```python
from build123d import *

# Parameters (mm, degrees)
SKETCH1_W               = 45.72
SKETCH1_H               = 17.78
BOSS_EXTRUDE1_DEPTH     = 45.72
SKETCH2_W               = 38.1
SKETCH2_H               = 12.7
CUT_EXTRUDE1_DEPTH      = 41.91
SKETCH6_R               = 3.048
CUT_EXTRUDE2_DEPTH      = 9.328339826
CUT_EXTRUDE2_DEPTH_BACK = 15.24


with BuildPart() as part:
    # Sketch1 → Boss-Extrude1 (new body)
    with BuildSketch(Plane(origin=(0, 0, 0), x_dir=(1, 0, 0), z_dir=(0, 1, 0))):
        with Locations((22.86, 8.89)):
            Rectangle(SKETCH1_W, SKETCH1_H)
    extrude(amount=BOSS_EXTRUDE1_DEPTH)

    # Sketch2 → Cut-Extrude1 (cut)
    with BuildSketch(Plane(origin=(0, 45.72, 0), x_dir=(1, 0, 0), z_dir=(0, 1, 0))):
        with Locations((22.86, 8.89)):
            Rectangle(SKETCH2_W, SKETCH2_H)
    extrude(amount=-CUT_EXTRUDE1_DEPTH, mode=Mode.SUBTRACT)

    # Sketch6 → Cut-Extrude2 (cut, two sides)
    with BuildSketch(Plane(origin=(0, 0, 0), x_dir=(0.974501657, 0.176548089, -0.138482102), z_dir=(0.182159664, -0.982845594, 0.028851256))) as cut_extrude2_sk:
        with Locations((23.128298386, -5.852866773)):
            Circle(SKETCH6_R)
        with Locations((16.079712461, -6.800485078)):
            Circle(SKETCH6_R)
        with Locations((30.176884312, -4.905248468)):
            Circle(SKETCH6_R)
    extrude(amount=CUT_EXTRUDE2_DEPTH, mode=Mode.SUBTRACT)
    extrude(cut_extrude2_sk.sketch, amount=-CUT_EXTRUDE2_DEPTH_BACK, mode=Mode.SUBTRACT)


solid = part.part
```
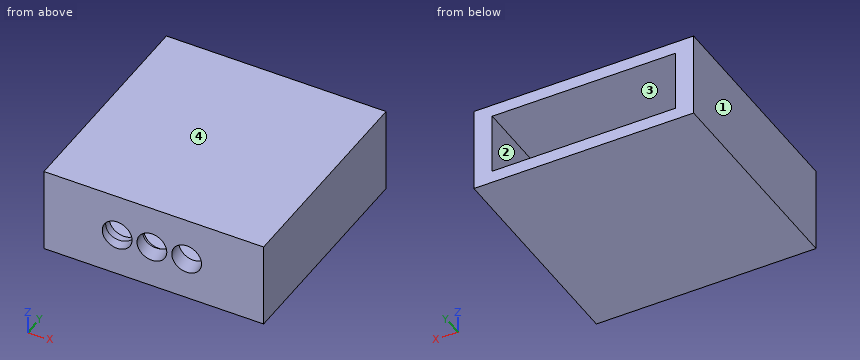
Model file for the job. Use its own axes, mm. Face numbers are marked on the shaded views. Coordinates: 2 decimals unless noted, no trailing zeros. Order: outer loops, then holes, each group sorted by start corner. A loop starts at its lowest first (then second) coordinate and runs counter-clockwise, first axis right, second up. Notation, with made-up numbers: (62, 11.25) - (95, 11.25) arc R12 cw to (95, 28.25) - close; hole circle Ø2 at (57, 84.25). An arc over 180 degrees is marked (long way). Return JSON: item names as keys, results as strings. Group by question number.
1) Saw through at A-A, the plane y = 42. Write the cut outline in (x, z).
2) Flat gauge pins, fed straight in: P1, Ø1, axis at x = 41, z = -3.5, coming from the -Y side; P2, Ø1, axis at x = 5.5, z = -4, coming from the +Y side. Where does each tip first touch, or does it go through?
3) Saw through at C-C, the plane z = -8.5. Count the separate pieces of the cut face and the enclosed holes in it, plus the area to 3 significant figures.
4) Saw through at B-B, the plane z = -13. Write the cut outline in (x, y), plus the area to 3 significant figures.
5) Mould opens along X. For the marked faces 1, 2, 3 and 4 say: released by +X, released by -X, zero draft, split by the parting line, or undercut.
6) Probe line 1 (Z direction, x = 7, y = 41.5); line 2 (X direction, y = 18, z = -10.5); line 3 (Y direction, x = 30, z = -12). List the from-to ranges inside material, lowest first. Write a range as from..to.
Values found:
{
 "1": {"outline": "(0, -17.78) - (45.72, -17.78) - (45.72, 0) - (0, 0) - close; hole (3.81, -15.24) - (41.91, -15.24) - (41.91, -2.54) - (3.81, -2.54) - close"},
 "2": {"P1": "stops at y = 0", "P2": "stops at y = 3.81"},
 "3": {"separate pieces": "4", "enclosed holes": "0", "area": "423 mm²"},
 "4": {"outline": "(0, 0) - (45.72, 0) - (45.72, 45.72) - (41.91, 45.72) - (41.91, 3.81) - (3.81, 3.81) - (3.81, 45.72) - (0, 45.72) - close", "area": "494 mm²"},
 "5": {"face 1": "released by -X", "face 2": "undercut", "face 3": "undercut", "face 4": "zero draft"},
 "6": {"line 1": "z = -17.78..-15.24, -2.54..0", "line 2": "x = 0..3.81, 41.91..45.72", "line 3": "y = 0..3.81"}
}
